The model under review builds one solid part; all positions refer to its coordinate system, in mm. A direction names the side the tool comes from. Round coordinates to 2 decimals unless told otherwise and drop trailing zeros. Loops run counter-clockwise (first coordinate to the right, second up) from the corner with the lowest first, then second, coordinate; pieces in that order, holes last. Notation, with made-up numbers: (44.5, 21.5) -> (100.5, 21.5) arc R6 cw to (100.5, 27.5) -> close; hole circle Ø11 at (-10, 37.5). An arc over 180 degrees is marked (long way). Use a Markdown table: item, result. Add a question column.
1) Wall thickness on probe 1 along X at (y, z) = (-4.9, 36); probe 2 along Z at (x, y) = (18.5, -1.25); probe 3 along X at (y, z) = (-5.7, -41): over which ranges is each line inside the solid? List them lowest first.
2) Insertion check: pin 1 (4 mm diameter, centred on x = 20.5, z = 79.5, fed in from -Y). The pin has a flat end and moves straight along its axis. Give the tip position at first contact, or say it passes through.
3) Consider section B-B on y = -3.9. Give the boundary of the cut face in (x, z).
4) Consider section C-C on x = 9.5. Give the boundary of the cut face in (y, z).
5) Mouldability with a two-part tool opening along Z and no side actions: class faces 3 (the flat face through (38.553, -3, 27)), 4 (the cylindrical face through (-7.19, -2.96, -26.96)), 5 (the flat face through (-11, -3, 133.044)) as released by +Z, released by -Z, zero draft, split by the parting line, or undercut.
6) Consider section A-A on z = 42.5. Give the boundary of the cut face in (x, y), plus the area to 3 significant figures.
7) For faces 1 (the flat face through (-30, -3, -23.956)), 2 (the cylindrical face through (35.7, -2.96, 130.04)), list the 3-axis set-ups (+Z, -Z, +X, -X, +Y, -Y) from which the entire face can be reached by the end or side of a thin tool; tool diameter is ignored.
from build123d import *

# Parameters (mm, degrees)
F1_DEPTH = 6


with BuildPart() as f1:
    # F0 (on Front) → F1 (new body)
    with BuildSketch(Plane.XZ):
        with BuildLine():
            Line((28.552629, 133.043638), (-51.447371, 133.043638))
            ThreePointArc((-51.447371, 133.043638), (-58.518439, 130.114706), (-61.447371, 123.043638))
            Line((-61.447371, 123.043638), (-61.447371, -66.956362))
            ThreePointArc((-61.447371, -66.956362), (-58.518439, -74.027429), (-51.447371, -76.956362))
            Line((-51.447371, -76.956362), (28.552629, -76.956362))
            ThreePointArc((28.552629, -76.956362), (35.623697, -74.027429), (38.552629, -66.956362))
            Line((38.552629, -66.956362), (38.552629, 123.043638))
            ThreePointArc((38.552629, 123.043638), (35.623697, 130.114706), (28.552629, 133.043638))
        make_face()
        with BuildLine():
            Line((-46.447371, -23.956362), (-46.447371, 118.043638))
            Line((-46.447371, 118.043638), (23.552629, 118.043638))
            Line((23.552629, 118.043638), (23.552629, -61.956362))
            Line((23.552629, -61.956362), (-4.337173, -61.956362))
            Line((-4.337173, -61.956362), (-4.337173, -33.956362))
            ThreePointArc((-4.337173, -33.956362), (-7.266106, -26.885294), (-14.337173, -23.956362))
            Line((-14.337173, -23.956362), (-46.447371, -23.956362))
        make_face(mode=Mode.SUBTRACT)
    extrude(amount=F1_DEPTH)


solid = f1.part
Result set:
| question | item | result |
|---|---|---|
| 1 | probe 1 | -61.45 to -46.45, 23.55 to 38.55 |
| 1 | probe 2 | -76.96 to -61.96, 118.04 to 133.04 |
| 1 | probe 3 | -61.45 to -4.34, 23.55 to 38.55 |
| 2 | pin 1 | through |
| 3 | outline | (-61.45, -66.96) arc R10 ccw to (-51.45, -76.96) -> (28.55, -76.96) arc R10 ccw to (38.55, -66.96) -> (38.55, 123.04) arc R10 ccw to (28.55, 133.04) -> (-51.45, 133.04) arc R10 ccw to (-61.45, 123.04) -> close; hole (-46.45, -23.96) -> (-14.34, -23.96) arc R10 cw to (-4.34, -33.96) -> (-4.34, -61.96) -> (23.55, -61.96) -> (23.55, 118.04) -> (-46.45, 118.04) -> close |
| 4 | outline | (-6, -76.96) -> (0, -76.96) -> (0, -61.96) -> (-6, -61.96) -> close; (-6, 118.04) -> (0, 118.04) -> (0, 133.04) -> (-6, 133.04) -> close |
| 5 | face 3 | zero draft |
| 5 | face 4 | undercut |
| 5 | face 5 | released by +Z |
| 6 | outline | (-61.45, -6) -> (-46.45, -6) -> (-46.45, 0) -> (-61.45, 0) -> close; (23.55, -6) -> (38.55, -6) -> (38.55, 0) -> (23.55, 0) -> close |
| 6 | area | 180 mm2 |
| 7 | face 1 | +Y, -Y |
| 7 | face 2 | +Z, +X, +Y, -Y |
